Part model, mm, in its own coordinate system. Face numbers are marked on the shaded views. A direction names the side the tool comes from. Give positions to 0.01 mm unless a question says otherwise; leave off trailing zeros. Write each loop counter-clockwise with the first axis right and the second up, starting at its lowest first coordinate (ties: lowest second). Pieces come first, ordered by that corner, then holes. Notation, with made-up numbers: M -10.5,-6.75 L 13.5,-6.75 A33 cw 13.5,22.25 Z; hole C -17,46 d11. An arc over 180 degrees is marked long. Answer as CSV lines item,"result". Start each with the question number.
1) Slice it at A-A, the plane y = 9.25. Give the cut face in (x, z), plus the area to 3 significant figures.
2) Tool access for the marked faces 4, 5 and 6: list every direction of +Z, -Z, +X, -X, +Y, -Y with a clear straight run to the whole face (end or side of a thin tool).
3) Wall check: line 1 along X through (y, z) = (9.5, -7.75); line 2 along X through (y, z) = (9.5, 8.5); line 3 along Y through (x, z) = (4, 9). Give the ranges that are in metal, low to high. Write a range as from..to.
4) Slice it at D-D, the plane y = 1.5. Give the cut face in (x, z).
5) Mould opens along X. For the marked faces 1, 2 and 3 say: pulls with the +X half, pulls with the -X half, needs draft (parallel to the pull), parting line crosses it, or undercut.
6) Slice it at C-C, the plane x = 11.5. Give the cut face in (y, z), plus the area to 3 significant figures.
7) Slice it at B-B, the plane z = 8.5. Give the cut face in (x, y).
8) Pin check, flat tips, straight feed: pin 1 Ø0.9 at (x, z) = (-13, 9.5) entering from +Y; pin 2 Ø1 at (y, z) = (3.5, 11.5) entering from -X; pin 3 Ø2 at (y, z) = (7, -6) entering from +X. Stop position of each tip, or through.
```python
from build123d import *

# Parameters (mm, degrees)
SKETCH1_W           = 28
SKETCH1_H           = 27
BOSS_EXTRUDE1_DEPTH = 14
SHELL1_T            = -2
SKETCH2_W           = 24
SKETCH2_H           = 23
SKETCH2_W_2         = 6
SKETCH2_H_2         = 1
BOSS_EXTRUDE2_DEPTH = 2.5
CUT_EXTRUDE1_REACH  = 35.481
SKETCH3_W           = 24
SKETCH3_H           = 9.5
CUT_EXTRUDE2_REACH  = 25.964
SKETCH4_R           = 1.6
BOSS_EXTRUDE3_DEPTH = 14
CUT_EXTRUDE4_REACH  = 34.368
SKETCH7_W           = 10
SKETCH7_H           = 8.6
SKETCH8_R           = 3.6
CUT_EXTRUDE5_DEPTH  = 1.5
FILLET1_R           = 0.5


with BuildPart() as part:
    # Sketch1 → Boss-Extrude1 (new body)
    with BuildSketch(Plane(origin=(0, 0, 0), x_dir=(1, 0, 0), z_dir=(0, 1, 0))):
        Rectangle(SKETCH1_W, SKETCH1_H)
    extrude(amount=BOSS_EXTRUDE1_DEPTH)

    # Shell1
    shell1_openings = [part.faces().sort_by_distance(p)[0] for p in [
        (0, 14, 0),
    ]]
    offset(amount=SHELL1_T, openings=shell1_openings, kind=Kind.INTERSECTION)

    # Sketch2 → Boss-Extrude2 (add)
    with BuildSketch(Plane(origin=(0, 2, 0), x_dir=(1, 0, 0), z_dir=(0, 1, 0))):
        Rectangle(SKETCH2_W, SKETCH2_H)
        with Locations((0, 6.25)):
            Rectangle(SKETCH2_W_2, SKETCH2_H_2, mode=Mode.SUBTRACT)
    extrude(amount=BOSS_EXTRUDE2_DEPTH)

    # Sketch3 → Cut-Extrude1 (cut, up to next)
    with BuildSketch(Plane.XY.offset(13.5), mode=Mode.PRIVATE) as cut_extrude1_sk1:
        with Locations((0, 9.25)):
            Rectangle(SKETCH3_W, SKETCH3_H)
    cut_extrude1_tool1 = extrude(cut_extrude1_sk1.sketch, amount=-CUT_EXTRUDE1_REACH, mode=Mode.PRIVATE) & part.part
    add(cut_extrude1_tool1.solids().sort_by_distance((0, 9.25, 13.5))[0], mode=Mode.SUBTRACT)

    # Sketch4 → Cut-Extrude2 (cut, up to next)
    with BuildSketch(Plane(origin=(0, 14, 0), x_dir=(1, 0, 0), z_dir=(0, 1, 0)), mode=Mode.PRIVATE) as cut_extrude2_sk1:
        with Locations(Location((-11.5, -8.5, 0), (0, 0, 251.790043136))):
            Circle(SKETCH4_R)
    cut_extrude2_tool1 = extrude(cut_extrude2_sk1.sketch, amount=-CUT_EXTRUDE2_REACH, mode=Mode.PRIVATE) & part.part
    # Sketch4 → Cut-Extrude2 (cut, up to next)
    with BuildSketch(Plane(origin=(0, 14, 0), x_dir=(1, 0, 0), z_dir=(0, 1, 0)), mode=Mode.PRIVATE) as cut_extrude2_sk2:
        with Locations(Location((11.5, -8.5, 0), (0, 0, 288.209956864))):
            Circle(SKETCH4_R)
    cut_extrude2_tool2 = extrude(cut_extrude2_sk2.sketch, amount=-CUT_EXTRUDE2_REACH, mode=Mode.PRIVATE) & part.part
    add(cut_extrude2_tool1.solids().sort_by_distance((-11.5, 14, 8.5))[0], mode=Mode.SUBTRACT)
    add(cut_extrude2_tool2.solids().sort_by_distance((11.5, 14, 8.5))[0], mode=Mode.SUBTRACT)

    # Sketch5 → Boss-Extrude3 (add)
    with BuildSketch(Plane(origin=(0, 14, 0), x_dir=(1, 0, 0), z_dir=(0, 1, 0))):
        with BuildLine():
            Line((12, -4.980131585), (12, -6.980131585))
            ThreePointArc((12, -6.980131585), (13.1, -8.5), (12, -10.019868415))
            Line((12, -10.019868415), (12, -12.019868415))
            ThreePointArc((12, -12.019868415), (15.055203744, -8.5), (12, -4.980131585))
        make_face()
        with BuildLine():
            Line((-12, -4.980131585), (-12, -6.980131585))
            ThreePointArc((-12, -6.980131585), (-13.1, -8.5), (-12, -10.019868415))
            Line((-12, -10.019868415), (-12, -12.019868415))
            ThreePointArc((-12, -12.019868415), (-15.055203744, -8.5), (-12, -4.980131585))
        make_face()
    extrude(amount=-BOSS_EXTRUDE3_DEPTH)

    # Sketch7 → Cut-Extrude4 (cut, up to next)
    with BuildSketch(Plane.XY.offset(-11.5), mode=Mode.PRIVATE) as cut_extrude4_sk1:
        with Locations((0, 9.7)):
            Rectangle(SKETCH7_W, SKETCH7_H)
    cut_extrude4_tool1 = extrude(cut_extrude4_sk1.sketch, amount=-CUT_EXTRUDE4_REACH, mode=Mode.PRIVATE) & part.part
    add(cut_extrude4_tool1.solids().sort_by_distance((0, 9.7, -11.5))[0], mode=Mode.SUBTRACT)

    # Sketch8 → Cut-Extrude5 (cut)
    with BuildSketch(Plane(origin=(0, 14, 0), x_dir=(1, 0, 0), z_dir=(0, 1, 0))):
        with Locations((11.5, -8.5)):
            Circle(SKETCH8_R)
        with Locations((-11.5, -8.5)):
            Circle(SKETCH8_R)
    extrude(amount=-CUT_EXTRUDE5_DEPTH, mode=Mode.SUBTRACT)

    # Fillet1
    fillet1_edges = [part.edges().sort_by_distance(p)[0] for p in [
        (14, 14, 12.295183385),
        (9.5, 14, -13.5),
        (-13, 14, 13.5),
        (-14, 14, -3.795183385),
        (14, 14, -3.795183385),
        (-14, 14, 12.295183385),
        (13, 14, 13.5),
        (-14, 7, 13.5),
        (14, 7, 13.5),
        (-9.5, 14, -13.5),
    ]]
    fillet(fillet1_edges, radius=FILLET1_R)


solid = part.part
```
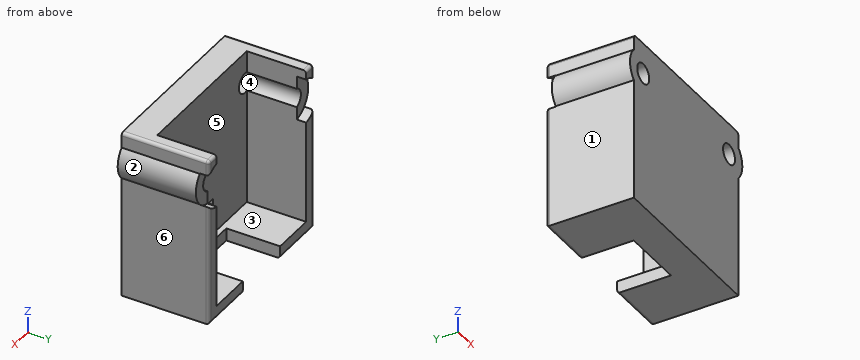
Found:
1,outline,"M -14,-13.5 L -5,-13.5 L -5,-11.5 L -12,-11.5 L -12,6.98 A1.6 cw -12,10.02 L -12,13.5 L -13.5,13.5 A0.5 ccw -14,13 L -14,11.03 A3.56 ccw -14,5.97 Z; M 5,-13.5 L 14,-13.5 L 14,5.97 A3.56 ccw 14,11.03 L 14,13 A0.5 ccw 13.5,13.5 L 12,13.5 L 12,10.02 A1.6 cw 12,6.98 L 12,-11.5 L 5,-11.5 Z"
1,area,"138 mm²"
2,face 4,"+Y, -Y"
2,face 5,"+Z, +Y"
2,face 6,"-Z, +X, +Y, -Y"
3,line 1,"-14..-12, 12..14"
3,line 2,"-15.06..-13.1, 13.1..15.06"
3,line 3,"0..4.5"
4,outline,"M -14,-13.5 L 14,-13.5 L 14,5.97 A3.56 ccw 14,11.03 L 14,13 A0.5 ccw 13.5,13.5 L -13.5,13.5 A0.5 ccw -14,13 L -14,11.03 A3.56 ccw -14,5.97 Z; hole C -11.5,8.5 d3.2; hole C 11.5,8.5 d3.2"
5,face 1,"pulls with the -X half"
5,face 2,"pulls with the +X half"
5,face 3,"undercut"
6,outline,"M 0,-13.5 L 13.5,-13.5 A0.5 ccw 14,-13 L 14,-11.5 L 4.5,-11.5 L 4.5,6.9 L 0,6.9 Z; M 0,10.1 L 4.5,10.1 L 4.5,13.5 L 0,13.5 Z"
6,area,"126 mm²"
7,outline,"M -15.06,0 L -13.1,0 L -13.1,12.5 L -15.06,12.5 Z; M -9.9,0 L 9.9,0 L 9.9,4.5 L -9.9,4.5 Z; M 13.1,0 L 15.06,0 L 15.06,12.5 L 13.1,12.5 Z"
8,pin 1,"y = 12.5"
8,pin 2,"x = -14.03"
8,pin 3,"x = 14"
